Autodesk Inventor part; units mm, degrees
ref_plane "YZ Plane" through (0, 0, 0) normal (1, 0, 0) x (0, 1, 0)
ref_plane "XZ Plane" through (0, 0, 0) normal (0, 1, 0) x (-1, 0, 0)
ref_plane "XY Plane" through (0, 0, 0) normal (0, 0, 1) x (1, 0, 0)
sketch "Sketch1" plane through (0, 0, 0) normal (0, 1, 0) x (-1, 0, 0)
  line L0 (0, 0) -> (20, 0)
  line L1 (20, 0) -> (20, -99.7)
  line L2 (20, -99.7) -> (0, -99.7)
  line L3 (0, -99.7) -> (0, 0)
  line L4 (0, 0) -> (5, 0)
  line L5 (5, 0) -> (5, -4)
  line L6 (5, -4) -> (0, -4)
  line L7 (0, -4) -> (0, 0)
  line L8 (0, -99.7) -> (5, -99.7)
  line L9 (5, -99.7) -> (5, -95.7)
  line L10 (5, -95.7) -> (0, -95.7)
  line L11 (0, -95.7) -> (0, -99.7)
  line L12 (5, -4) -> (15, -4)
  line L13 (5, -95.7) -> (15, -95.7)
  circle A0 centre (15, -4) radius 2
  circle A1 centre (5, -4) radius 2
  circle A2 centre (15, -95.7) radius 2
  circle A3 centre (5, -95.7) radius 2
  dimension "d0" = 20
  dimension "d1" = 99.7
  dimension "d2" = 5
  dimension "d3" = 4
  dimension "d4" = 5
  dimension "d5" = 4
  dimension "d6" = 10
  dimension "d7" = 10
  dimension "d8" = 4
  dimension "d9" = 4
  dimension "d10" = 4
  dimension "d11" = 4
extrude "Extrusion1" add sketch "Sketch1" along normal blind 4 contours L0 L5 A1 L6 L3 | L0 L1 L2 L9 A3 L10 L3 L6 A1 L5 | L10 A3 L9 L2 L3
sketch "Sketch2" plane through (0, 4, 0) normal (0, 1, 0) x (1, 0, 0)
  line L0 (-20, 99.7) -> (-20, 0)
  line L1 (0, 0) -> (0, 99.7)
  line L2 (-20, 0) -> (0, 0)
  line L3 (0, 0) -> (0, 8)
  line L4 (0, 8) -> (-20, 8)
  line L5 (-20, 8) -> (-20, 0)
  line L6 (0, 99.7) -> (-20, 99.7)
  line L7 (-20, 99.7) -> (0, 99.7)
  line L8 (0, 99.7) -> (0, 91.7)
  line L9 (0, 91.7) -> (-20, 91.7)
  line L10 (-20, 91.7) -> (-20, 99.7)
  line L11 (-20, 91.7) -> (0, 91.7)
  line L12 (0, 91.7) -> (0, 8)
  line L13 (0, 8) -> (-20, 8)
  line L14 (-20, 8) -> (-20, 91.7)
  dimension "d14" = 8
  dimension "d15" = 8
sketch "Sketch3" plane through (0, 4, 0) normal (0, 1, 0) x (1, 0, 0)
  point P0 (0, 0)
extrude "Extrusion2" cut sketch "Sketch2" against normal blind 2 contours L9 L1 L4 L0
sketch "Sketch4" plane through (0, 2, 0) normal (0, 1, 0) x (1, 0, 0)
  line L0 (-20, 8) -> (-20, 91.7)
  line L1 (-20, 49.85) -> (-10, 49.85)
  line L2 (-13.75, 19.85) -> (-6.25, 19.85)
  line L3 (-6.25, 19.85) -> (-6.25, 79.85)
  line L4 (-6.25, 79.85) -> (-13.75, 79.85)
  line L5 (-13.75, 79.85) -> (-13.75, 19.85)
  line L6 (-13.75, 19.85) -> (-6.25, 79.85) construction
  line L7 (-6.25, 19.85) -> (-13.75, 79.85) construction
  point P0 (0, 0)
  dimension "d18" = 10
  dimension "d19" = 7.5
  dimension "d20" = 60
extrude "Extrusion3" cut sketch "Sketch4" against normal blind 2
properties part number "servo2servo_support"
Model file for the job. Use its own axes, mm. A direction names the side the tool comes from. Coordinates: 2 decimals unless noted, no trailing zeros. Loops run counter-clockwise (first coordinate to the right, second up) from the corner with the lowest first, then second, coordinate; pieces in that order, holes last. Notation, with made-up numbers: (23, 28) -> (32, 28) arc R16 cw to (32, 54) -> close; hole circle Ø5 at (70.25, -16.5). An arc over 180 degrees is marked (long way). Answer as a JSON object with one key per item and string values.
Q1. Cut at B-B (y = 3.25). List the corners of the cut face in (x, z), and give its area (3 significant figures).
Report:
{"outline": "(-20, -99.7) -> (0, -99.7) -> (0, -91.7) -> (-20, -91.7) -> close; (-20, -8) -> (0, -8) -> (0, 0) -> (-20, 0) -> close; hole circle Ø4 at (-15, -95.7); hole circle Ø4 at (-15, -4); hole circle Ø4 at (-5, -95.7); hole circle Ø4 at (-5, -4)", "area": "270 mm2"}
Q2. Cut at A-A (x = -15). List the corners of the cut face in (y, z).
Report:
{"outline": "(0, -99.7) -> (4, -99.7) -> (4, -97.7) -> (0, -97.7) -> close; (0, -93.7) -> (4, -93.7) -> (4, -91.7) -> (2, -91.7) -> (2, -8) -> (4, -8) -> (4, -6) -> (0, -6) -> close; (0, -2) -> (4, -2) -> (4, 0) -> (0, 0) -> close"}
Q3. Flat gauge pins, fed straight in: P1, Ø1, axis at x = -12, y = 1.5, coming from the +Z side; P2, Ø2, axis at x = -8, z = -40, coming from the -Y side; P3, Ø10, axis at x = -16, z = -82.5, coming from the +Y side. Where does each tip first touch, or does it go through?
Report:
{"P1": "stops at z = 0", "P2": "passes through", "P3": "stops at y = 2"}
Q4. Probe probe 1 along Z at (x, y) = (-15, 1.4); probe 2 along Z at (x, y) = (-15, 2.9); probe 3 along X at (y, z) = (2.35, -4). List the from-to ranges inside material, lowest first.
Report:
{"probe 1": "z = -99.7 to -97.7, -93.7 to -6, -2 to 0", "probe 2": "z = -99.7 to -97.7, -93.7 to -91.7, -8 to -6, -2 to 0", "probe 3": "x = -20 to -17, -13 to -7, -3 to 0"}
Q5. Cut at C-C (z = -95.7). List the corners of the cut face in (x, y), and give its area (3 significant figures).
Report:
{"outline": "(-20, 0) -> (-17, 0) -> (-17, 4) -> (-20, 4) -> close; (-13, 0) -> (-7, 0) -> (-7, 4) -> (-13, 4) -> close; (-3, 0) -> (0, 0) -> (0, 4) -> (-3, 4) -> close", "area": "48.0 mm2"}
Q6. Pull direction Z, two halves, no side cores. Call faces 1 (the flat face through (-10, 2, -99.7)), 2 (the flat face through (-10, 3, -8)), 3 (the flat face through (-10, 4, -4)): released by +Z, released by -Z, zero draft, split by the parting line, or undercut.
Report:
{"face 1": "released by -Z", "face 2": "undercut", "face 3": "zero draft"}
Q7. 3-axis set-ups, long thin cutter, end or side, ignore diameter. For faces 4 (the flat face through (-10, 1, -79.85)), 5 (the flat face through (-14, 0, -49)), 6 (the flat face through (-10, 3, -91.7)): which of +Z, -Z, +X, -X, +Y, -Y reach the whole face in a straight line?
Report:
{"face 4": "+Y, -Y", "face 5": "+Z, -Z, +X, -X, -Y", "face 6": "+X, -X, +Y"}
Q8. Cut at D-D (x = -10.25). List the corners of the cut face in (y, z), and give its area (3 significant figures).
Report:
{"outline": "(0, -99.7) -> (4, -99.7) -> (4, -91.7) -> (2, -91.7) -> (2, -79.85) -> (0, -79.85) -> close; (0, -19.85) -> (2, -19.85) -> (2, -8) -> (4, -8) -> (4, 0) -> (0, 0) -> close", "area": "111 mm2"}
